from build123d import *

# Parameters (mm, degrees)
SKIZZE1_W                       = 200
SKIZZE1_H                       = 50
AUFSATZ_LINEAR_AUSTRAGEN1_DEPTH = 4
SKIZZE2_W                       = 15.5
SKIZZE2_H                       = 4
AUFSATZ_LINEAR_AUSTRAGEN2_DEPTH = 4
SCHNITT_LINEAR_AUSTRAGEN1_REACH = 6
SKIZZE4_W                       = 4
SKIZZE4_H                       = 15


with BuildPart() as part:
    # Skizze1 → Aufsatz-Linear austragen1 (new body)
    with BuildSketch(Plane.XY):
        with Locations((100, 25)):
            Rectangle(SKIZZE1_W, SKIZZE1_H)
    extrude(amount=AUFSATZ_LINEAR_AUSTRAGEN1_DEPTH)

    # Skizze2 → Aufsatz-Linear austragen2 (add)
    with BuildSketch(Plane(origin=(0, 0, 4), x_dir=(-1, 0, 0), z_dir=(0, 0, -1))):
        with Locations((-174.8, -2)):
            Rectangle(SKIZZE2_W, SKIZZE2_H)
        with Locations((-124.8, -2)):
            Rectangle(SKIZZE2_W, SKIZZE2_H)
        with Locations((-74.8, -2)):
            Rectangle(SKIZZE2_W, SKIZZE2_H)
        with Locations((-24.8, -2)):
            Rectangle(SKIZZE2_W, SKIZZE2_H)
    extrude(amount=AUFSATZ_LINEAR_AUSTRAGEN2_DEPTH)

    # Skizze4 → Schnitt-Linear austragen1 (cut, up to next)
    with BuildSketch(Plane.XY.offset(4), mode=Mode.PRIVATE) as schnitt_linear_austragen1_sk1:
        with Locations((2, 25)):
            Rectangle(SKIZZE4_W, SKIZZE4_H)
    schnitt_linear_austragen1_tool1 = extrude(schnitt_linear_austragen1_sk1.sketch, amount=-SCHNITT_LINEAR_AUSTRAGEN1_REACH, mode=Mode.PRIVATE) & part.part
    add(schnitt_linear_austragen1_tool1.solids().sort_by_distance((2, 25, 4))[0], mode=Mode.SUBTRACT)
    # Skizze4 → Schnitt-Linear austragen1 (cut, up to next)
    with BuildSketch(Plane.XY.offset(4), mode=Mode.PRIVATE) as schnitt_linear_austragen1_sk2:
        with Locations((198, 25)):
            Rectangle(SKIZZE4_W, SKIZZE4_H)
    schnitt_linear_austragen1_tool2 = extrude(schnitt_linear_austragen1_sk2.sketch, amount=-SCHNITT_LINEAR_AUSTRAGEN1_REACH, mode=Mode.PRIVATE) & part.part
    add(schnitt_linear_austragen1_tool2.solids().sort_by_distance((198, 25, 4))[0], mode=Mode.SUBTRACT)


solid = part.part
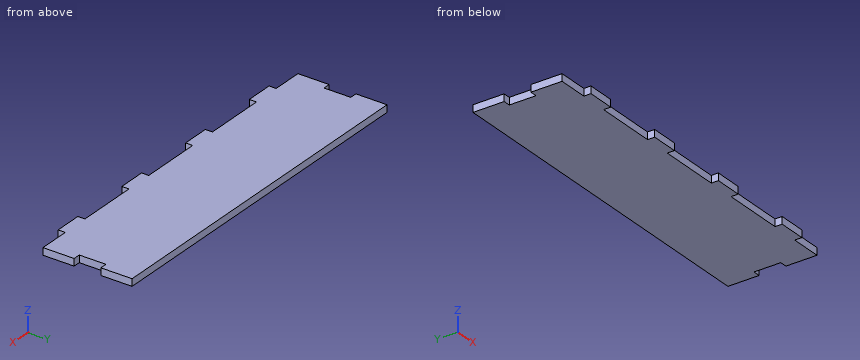
Geometry check sheet. Reference: the model listing, model coordinates, mm. Round coordinates to 2 decimals unless told otherwise and drop trailing zeros. Order: outer loops, then holes, each group sorted by start corner. A loop starts at its lowest first (then second) coordinate and runs counter-clockwise, first axis right, second up. Notation, with made-up numbers: M 27.5,-26 L 64.5,-26 A17 cw 64.5,5 Z; hole C 33.5,-39 d5. An arc over 180 degrees is marked long. Answer in a Markdown table with one row per item. Add a question column.
Item 1: Sectioned sample at C-C, the plane y = 27.5. Enter the section's corners in (x, z), plus the area to 3 significant figures.
Item 2: Sectioned sample at A-A, the plane z = 2.4. Enter the section's corners in (x, y), plus the area to 3 significant figures.
Item 3: Depth check by flat-ended pin: pin 1 Ø2 at (y, z) = (-2, 2.5) entering from +X; pin 2 Ø1.2 at (y, z) = (-2, 1) entering from -X; pin 3 Ø2 at (x, z) = (99.5, 3) entering from -Y; pin 4 Ø1 at (x, y) = (75.5, 32) entering from -Z. Enter the tip coordinate at first touch or a pass-through.
Item 4: Sectioned sample at B-B, the plane x = 48.5. Enter the section's corners in (y, z), plus the area to 3 significant figures.
Item 5: Material ranges on L1, parallel to X at y = 30, z = 2.3; L2, parallel to Y at x = 133.5, z = 3.5, recorded low to high. Write a range as [from, to].
Filled in:
| question | item | result |
|---|---|---|
| 1 | outline | M 4,0 L 196,0 L 196,4 L 4,4 Z |
| 1 | area | 768 mm² |
| 2 | outline | M 0,0 L 17.05,0 L 17.05,-4 L 32.55,-4 L 32.55,0 L 67.05,0 L 67.05,-4 L 82.55,-4 L 82.55,0 L 117.05,0 L 117.05,-4 L 132.55,-4 L 132.55,0 L 167.05,0 L 167.05,-4 L 182.55,-4 L 182.55,0 L 200,0 L 200,17.5 L 196,17.5 L 196,32.5 L 200,32.5 L 200,50 L 0,50 L 0,32.5 L 4,32.5 L 4,17.5 L 0,17.5 Z |
| 2 | area | 10,100 mm² |
| 3 | pin 1 | stops at x = 182.55 |
| 3 | pin 2 | stops at x = 17.05 |
| 3 | pin 3 | stops at y = 0 |
| 3 | pin 4 | stops at z = 0 |
| 4 | outline | M 0,0 L 50,0 L 50,4 L 0,4 Z |
| 4 | area | 200 mm² |
| 5 | L1 | x = [4, 196] |
| 5 | L2 | y = [0, 50] |
